Could you check a few things on this model? Use its own coordinates, in mm. Coordinates: 2 decimals unless noted, no trailing zeros. Write each loop counter-clockwise with the first axis right and the second up, starting at its lowest first coordinate (ties: lowest second). Pieces come first, ordered by that corner, then holes.
```python
from build123d import *

# Parameters (mm, degrees)
SKETCH2_R               = 19.05
SKETCH2_R_2             = 12.954
BOSS_EXTRUDE1_DEPTH     = 685.8
CUT_EXTRUDE1_REACH      = 688.329
SKETCH3_W               = 50.8
SKETCH3_H               = 101.6
CUT_EXTRUDE2_REACH      = 688.329
CUT_EXTRUDE2_END_RADIUS = 19.05
SKETCH4_W               = 16.51
SKETCH4_H               = 38.1


with BuildPart() as part:
    # Sketch2 → Boss-Extrude1 (new body)
    with BuildSketch(Plane.XY):
        Circle(SKETCH2_R)
        Circle(SKETCH2_R_2, mode=Mode.SUBTRACT)
    extrude(amount=BOSS_EXTRUDE1_DEPTH)

    # Sketch3 → Cut-Extrude1 (cut, up to next)
    with BuildSketch(Plane(origin=(0, 0, 0), x_dir=(1, 0, 0), z_dir=(0, 1, 0)), mode=Mode.PRIVATE) as cut_extrude1_sk1:
        with Locations((0, -88.9)):
            Rectangle(SKETCH3_W, SKETCH3_H)
    cut_extrude1_tool1 = extrude(cut_extrude1_sk1.sketch, amount=CUT_EXTRUDE1_REACH, mode=Mode.PRIVATE) & part.part
    add(cut_extrude1_tool1.solids().sort_by_distance((0, 0, 88.9))[0], mode=Mode.SUBTRACT)

    # Cut-Extrude2: up to this cylinder (the profile starts inside it)
    cut_extrude2_end = Plane(origin=(0, 0, 463.55), z_dir=(0, 0, -1)) * Cylinder(CUT_EXTRUDE2_END_RADIUS, 1415.758, mode=Mode.PRIVATE)
    # Sketch4 → Cut-Extrude2 (cut, up to the surface)
    with BuildSketch(Plane(origin=(0, 0, 0), x_dir=(1, 0, 0), z_dir=(0, 1, 0)), mode=Mode.PRIVATE) as cut_extrude2_sk1:
        with Locations((4.699, -463.55)):
            Rectangle(SKETCH4_W, SKETCH4_H)
    cut_extrude2_tool1 = extrude(cut_extrude2_sk1.sketch, amount=CUT_EXTRUDE2_REACH, mode=Mode.PRIVATE) & cut_extrude2_end
    add(cut_extrude2_tool1.solids().sort_by_distance((4.699, 0, 463.55))[0], mode=Mode.SUBTRACT)


solid = part.part
```
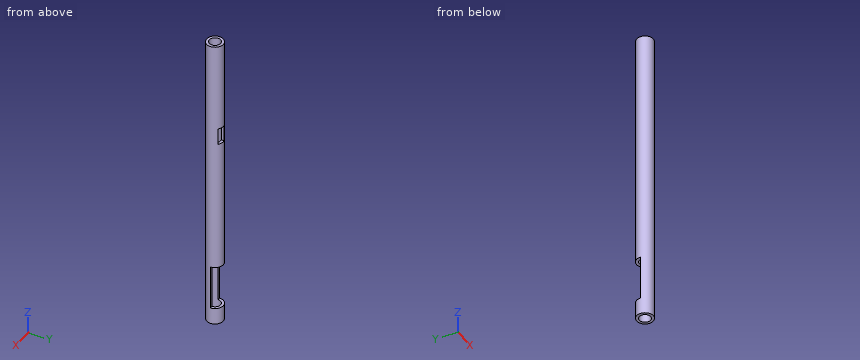
Item 1: I want a section at B-B, the plane z = 353. List the corners of the cut face in (x, y) for me, then the cut area to 3 significant figures.
Item 2: If I drill on line 1 along Y through (x, z) = (0, 361); line 2 along Z through (x, y) = (12, 9.5), over which ranges is the centre line in solid material (lowest first)?
Item 3: I want a section at A-A, the plane y = -7. List the corners of the cut face in (x, z) for me.
Item 4: Will these pins go through, and if not, where does the flat tip stop? pin 1 Ø5 at (x, z) = (16, 75.5) entering from +Y; pin 2 Ø12 at (y, z) = (6.5, 258) entering from +X; pin 3 Ø3 at (y, z) = (15.5, 460) entering from +X.
Taken from the geometry:
1. outline: circle Ø38.1 at (0, 0); hole circle Ø25.91 at (0, 0)
1. area: 613 mm2
2. line 1: y = -19.05 to -12.95, 12.95 to 19.05
2. line 2: z = 0 to 38.1, 139.7 to 444.5, 482.6 to 685.8
3. outline: (-17.72, 0) - (-10.9, 0) - (-10.9, 685.8) - (-17.72, 685.8) - close; (10.9, 0) - (17.72, 0) - (17.72, 685.8) - (10.9, 685.8) - close
4. pin 1: stops at y = 0
4. pin 2: stops at x = 19.04
4. pin 3: stops at x = -3.56
